For this review, take the finished solid that the model builds, in its own axes (mm). Give positions to 0.01 mm unless a question says otherwise; leave off trailing zeros. Order: outer loops, then holes, each group sorted by start corner. A loop starts at its lowest first (then second) coordinate and runs counter-clockwise, first axis right, second up.
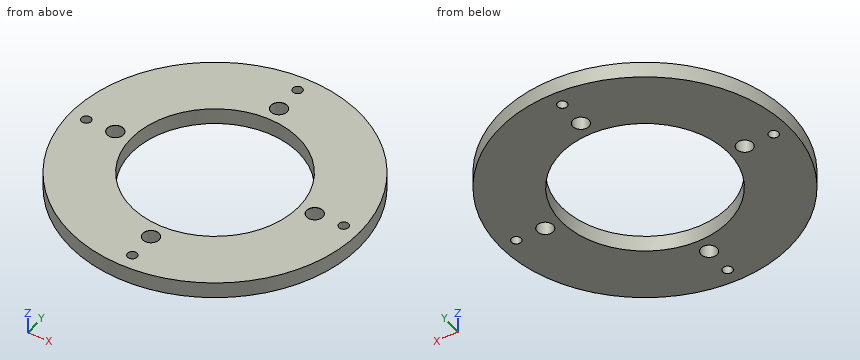
from build123d import *

# Parameters (mm, degrees)
SKETCH1_R                       = 45
SKETCH1_R_2                     = 26
BOSS_EXTRUDE1_DEPTH             = 5
F_5_0MM_DOWEL_HOLE1_D           = 5
F_5_0MM_DOWEL_HOLE1_CSINK_D     = 5.05
F_5_0MM_DOWEL_HOLE1_CSINK_ANGLE = 90
F_3_0MM_DOWEL_HOLE3_D           = 3
F_3_0MM_DOWEL_HOLE3_CSINK_D     = 3.05
F_3_0MM_DOWEL_HOLE3_CSINK_ANGLE = 90


with BuildPart() as part:
    # Sketch1 → Boss-Extrude1 (new body)
    with BuildSketch(Plane.XY):
        Circle(SKETCH1_R)
        Circle(SKETCH1_R_2, mode=Mode.SUBTRACT)
    extrude(amount=BOSS_EXTRUDE1_DEPTH)

    # Ø5.0mm Dowel Hole1 (through all)
    with Locations(Plane.XY.offset(5)):
        with Locations((0, 31), (-31, 0), (0, -31), (31, 0)):
            CounterSinkHole(F_5_0MM_DOWEL_HOLE1_D / 2, F_5_0MM_DOWEL_HOLE1_CSINK_D / 2, counter_sink_angle=F_5_0MM_DOWEL_HOLE1_CSINK_ANGLE)

    # Ø3.0mm Dowel Hole3 (through all)
    with Locations(Plane(origin=(0, 0, 0), x_dir=(-1, 0, 0), z_dir=(0, 0, -1))):
        with Locations((0, 40), (40, 0), (0, -40), (-40, 0)):
            CounterSinkHole(F_3_0MM_DOWEL_HOLE3_D / 2, F_3_0MM_DOWEL_HOLE3_CSINK_D / 2, counter_sink_angle=F_3_0MM_DOWEL_HOLE3_CSINK_ANGLE)


solid = part.part
1) We need section C-C on x = -40. Give the boundary of the cut face in (y, z) (3 decimals).
Answer sheet:
outline: (-20.616, 0) - (-1.525, 0) - (-1.5, 0.025) - (-1.5, 5) - (-20.616, 5) - close; (1.5, 0.025) - (1.525, 0) - (20.616, 0) - (20.616, 5) - (1.5, 5) - close
2) We need section D-D on y = 16. Give the boundary of the cut face in (x, z).
Answer sheet:
outline: (-42.06, 0) - (-20.49, 0) - (-20.49, 5) - (-42.06, 5) - close; (20.49, 0) - (42.06, 0) - (42.06, 5) - (20.49, 5) - close
3) We need section A-A on y = 0. Count the separate pieces of the cut face and the enclosed holes in it, then the cut area to 3 significant figures.
Answer sheet:
separate pieces: 6
enclosed holes: 0
area: 110 mm2
4) To check wall thickness, follow line 1 (Y direction, x = 0, z = 1.9); line 2 (Y direction, x = 1, z = 2.8); line 3 (Y direction, x = -33, z = 1.7). State the ranges of each line that lie inside material, in increasing order.
Answer sheet:
line 1: y = -45 to -41.5, -38.5 to -33.5, -28.5 to -26, 26 to 28.5, 33.5 to 38.5, 41.5 to 45
line 2: y = -44.99 to -41.12, -38.88 to -33.29, -28.71 to -25.98, 25.98 to 28.71, 33.29 to 38.88, 41.12 to 44.99
line 3: y = -30.59 to -1.5, 1.5 to 30.59
5) Clearance check with flat-ended pins moving along their axes: pin 1 (2.5 mm diameter, centred on x = 0, y = 40, fed in from +Z); pin 2 (6 mm diameter, centred on x = 31, y = 0, fed in from -Z); pin 3 (1.5 mm diameter, centred on x = 32, z = 4.5, fed in from -Y); pin 4 (3 mm diameter, centred on y = 17, z = 3, fed in from -X). State where each tip first meets the part, or that it passes through.
Answer sheet:
pin 1: passes through
pin 2: stops at z = 0
pin 3: stops at y = -32.38
pin 4: stops at x = -42.25
